from build123d import *

# Parameters (mm, degrees)
F0_W     = 50.8
F0_H     = 38.1
F1_DEPTH = 31.75
F3_DEPTH = 50.8
F4_W     = 25.4
F4_H     = 14.567647
F5_DEPTH = 25.4


with BuildPart() as f1:
    # F0 (on Front) → F1 (new body)
    with BuildSketch(Plane.XZ):
        with Locations((25.4, 19.05)):
            Rectangle(F0_W, F0_H)
    extrude(amount=F1_DEPTH)

    # F2 (on face) → F3 (cut)
    with BuildSketch(Plane.YZ.offset(50.8)):
        with BuildLine():
            Line((-31.75, 38.1), (-31.75, 12.7))
            ThreePointArc((-31.75, 12.7), (-16.061294, 22.411294), (-6.35, 38.1))
            Line((-6.35, 38.1), (-31.75, 38.1))
        make_face()
    extrude(amount=-F3_DEPTH, mode=Mode.SUBTRACT)

    # F4 (on face) → F5 (cut)
    with BuildSketch(Plane(origin=(0, 0, 0), x_dir=(-1, 0, 0), z_dir=(0, 1, 0))):
        with Locations((-25.4, 30.816177)):
            Rectangle(F4_W, F4_H)
    extrude(amount=-F5_DEPTH, mode=Mode.SUBTRACT)


solid = f1.part
Geometry check sheet. Reference: the model listing, model coordinates, mm. A direction names the side the tool comes from. Give positions to 0.01 mm unless a question says otherwise; leave off trailing zeros. Order: outer loops, then holes, each group sorted by start corner. A loop starts at its lowest first (then second) coordinate and runs counter-clockwise, first axis right, second up. Notation, with made-up numbers: (48, 4.25) - (98, 4.25) arc R18 cw to (98, 30.25) - close; hole circle Ø9 at (-19, 28). An arc over 180 degrees is marked (long way). Use one line per item in the form item = value.
1) Sectioned sample at A-A (z = 27). Record the boundary of the cut face in (x, y), and give its area (3 significant figures).
Working result:
outline = (0, -12.12) - (12.7, -12.12) - (12.7, 0) - (0, 0) - close; (38.1, -12.12) - (50.8, -12.12) - (50.8, 0) - (38.1, 0) - close
area = 308 mm^2
2) Material ranges on probe 1 along Z at (x, y) = (26, -3); probe 2 along Z at (x, y) = (4.5, -11.5); probe 3 along Y at (x, z) = (40, 32.5), recorded low to high. Write a range as from..to.
Working result:
probe_1 = 0..23.53
probe_2 = 0..27.86
probe_3 = -8.71..0
3) Sectioned sample at B-B (y = -2). Record the boundary of the cut face in (x, z).
Working result:
outline = (0, 0) - (50.8, 0) - (50.8, 38.1) - (38.1, 38.1) - (38.1, 23.53) - (12.7, 23.53) - (12.7, 38.1) - (0, 38.1) - close
4) Depth check by flat-ended pin: pin 1 Ø1 at (x, y) = (22, -15) entering from +Z; pin 2 Ø5 at (x, z) = (32.5, 25.5) entering from -Y; pin 3 Ø12 at (x, y) = (36, -25) entering from -Z; pin 4 Ø2 at (x, y) = (17.5, -27.5) entering from +Z. Enter the tip coordinate at first touch or a pass-through.
Working result:
pin_1 = 23.53
pin_2 = -15.48
pin_3 = 0
pin_4 = 14.88
5) Sectioned sample at D-D (x = 8.5). Record the boundary of the cut face in (y, z).
Working result:
outline = (-31.75, 0) - (0, 0) - (0, 38.1) - (-6.35, 38.1) arc R40.27 cw to (-31.75, 12.7) - close
6) Access from +Z, -Z, +X, -X, +Y, -Y to the whole of each face (thin tool, end or side, straight path). Record for faces 1 (the face through (25, -31.75, 6)), 2 (the face through (26, -7, 23.532)).
Working result:
face_1 = +Z, -Z, +X, -X, -Y
face_2 = +Z, +Y, -Y
7) Sectioned sample at C-C (x = 27). Record the boundary of the cut face in (y, z).
Working result:
outline = (-31.75, 0) - (0, 0) - (0, 23.53) - (-14.98, 23.53) arc R40.27 cw to (-31.75, 12.7) - close
